The listing builds one solid part. Answer for the finished solid, in the listing's coordinates (mm). Face numbers are marked on the shaded views. A direction names the side the tool comes from. Give positions to 0.01 mm unless a question says otherwise; leave off trailing zeros. Order: outer loops, then holes, each group sorted by start corner. A loop starts at its lowest first (then second) coordinate and runs counter-clockwise, first axis right, second up. Notation, with made-up numbers: (14, 80) -> (46, 80) arc R25 ccw to (46, 110) -> close; hole circle Ø3 at (88.25, 75.5). An arc over 180 degrees is marked (long way). Answer as a JSON object with one key per item and string values. Group by question number.
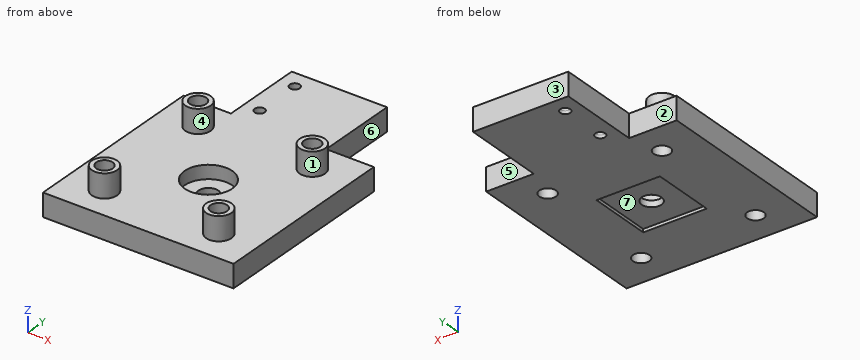
```python
from build123d import *

# Parameters (mm, degrees)
SKETCH1_W           = 38.1
SKETCH1_H           = 76.2
BOSS_EXTRUDE1_DEPTH = 7.9375
SKETCH2_R           = 3.96875
CUT_EXTRUDE1_DEPTH  = 44.330317403
SKETCH4_R           = 9.525
CUT_EXTRUDE2_DEPTH  = 5.3975
SKETCH8_W           = 19.05
SKETCH8_H           = 76.2
BOSS_EXTRUDE5_DEPTH = 7.9375
SKETCH5_R           = 5.08
BOSS_EXTRUDE2_DEPTH = 9.4488
SKETCH6_R           = 3.302
CUT_EXTRUDE3_DEPTH  = 57.617165486
SKETCH7_W           = 38.1
SKETCH7_H           = 33.02
SKETCH7_R           = 2
BOSS_EXTRUDE4_DEPTH = 7.9375
SKETCH9_R           = 3.302
SKETCH9_R_2         = 2
SKETCH9_W           = 25.4
SKETCH9_H           = 25.4
BOSS_EXTRUDE6_DEPTH = 1.27


with BuildPart() as part:
    # Sketch1 → Boss-Extrude1 (new body)
    with BuildSketch(Plane.XY):
        Rectangle(SKETCH1_W, SKETCH1_H)
    extrude(amount=BOSS_EXTRUDE1_DEPTH)

    # Sketch2 → Cut-Extrude1 (cut, through all)
    with BuildSketch(Plane.XY.offset(7.9375)):
        Circle(SKETCH2_R)
    extrude(amount=-CUT_EXTRUDE1_DEPTH, mode=Mode.SUBTRACT)

    # Sketch4 → Cut-Extrude2 (cut)
    with BuildSketch(Plane.XY.offset(7.9375)):
        Circle(SKETCH4_R)
    extrude(amount=-CUT_EXTRUDE2_DEPTH, mode=Mode.SUBTRACT)

    # Sketch8 → Boss-Extrude5 (add)
    with BuildSketch(Plane.XY.offset(7.9375)):
        with Locations((-28.575, 0)):
            Rectangle(SKETCH8_W, SKETCH8_H)
        with Locations((28.575, 0)):
            Rectangle(SKETCH8_W, SKETCH8_H)
    extrude(amount=-BOSS_EXTRUDE5_DEPTH)

    # Sketch5 → Boss-Extrude2 (add)
    with BuildSketch(Plane.XY.offset(7.9375)):
        with Locations(Location((22.86, 25.4, 0), (0, 0, 180))):
            Circle(SKETCH5_R)
        with Locations(Location((-22.86, 25.4, 0), (0, 0, 180))):
            Circle(SKETCH5_R)
    boss_extrude2 = extrude(amount=BOSS_EXTRUDE2_DEPTH)

    # Sketch6 → Cut-Extrude3 (cut, through all)
    with BuildSketch(Plane.XY.offset(17.3863)):
        with Locations((22.86, 25.4)):
            Circle(SKETCH6_R)
        with Locations(Location((-22.86, 25.4, 0), (0, 0, 180))):
            Circle(SKETCH6_R)
    cut_extrude3 = extrude(amount=-CUT_EXTRUDE3_DEPTH, mode=Mode.SUBTRACT)

    # Mirror1: Boss-Extrude2, Cut-Extrude3 across plane
    add(boss_extrude2.mirror(Plane.ZX))
    add(cut_extrude3.mirror(Plane.ZX), mode=Mode.SUBTRACT)

    # Sketch7 → Boss-Extrude4 (add)
    with BuildSketch(Plane.XY.offset(7.9375)):
        with Locations((0, 54.61)):
            Rectangle(SKETCH7_W, SKETCH7_H)
        with Locations((-12.7, 64.135)):
            Circle(SKETCH7_R, mode=Mode.SUBTRACT)
        with Locations(Location((-12.7, 45.085, 0), (0, 0, 180))):
            Circle(SKETCH7_R, mode=Mode.SUBTRACT)
    extrude(amount=-BOSS_EXTRUDE4_DEPTH)

    # Sketch9 → Boss-Extrude6 (add)
    with BuildSketch(Plane(origin=(0, 0, 0), x_dir=(-1, 0, 0), z_dir=(0, 0, -1))):
        Polygon((-19.05, 38.1), (-38.1, 38.1), (-38.1, -38.1), (38.1, -38.1), (38.1, 38.1), (19.05, 38.1), (19.05, 71.12), (-19.05, 71.12), align=None)
        with Locations(Location((-22.86, -25.4, 0), (0, 0, 180))):
            Circle(SKETCH9_R, mode=Mode.SUBTRACT)
        with Locations((22.86, -25.4)):
            Circle(SKETCH9_R, mode=Mode.SUBTRACT)
        with Locations((22.86, 25.4)):
            Circle(SKETCH9_R, mode=Mode.SUBTRACT)
        with Locations(Location((12.7, 64.135, 0), (0, 0, 180))):
            Circle(SKETCH9_R_2, mode=Mode.SUBTRACT)
        with Locations((12.7, 45.085)):
            Circle(SKETCH9_R_2, mode=Mode.SUBTRACT)
        with Locations(Location((-22.86, 25.4, 0), (0, 0, 180))):
            Circle(SKETCH9_R, mode=Mode.SUBTRACT)
        Rectangle(SKETCH9_W, SKETCH9_H, mode=Mode.SUBTRACT)
    extrude(amount=BOSS_EXTRUDE6_DEPTH)


solid = part.part
```
(1) A cutting plane is placed at B-B (x = 0). Determine the outline of the cut face in (y, z) (1 decimal).
(2) A cutting plane is placed at D-D (y = 25.4). Determine the outline of the cut face in (x, z).
(3) For a pull along X with two mould halves and no side action, classify the marked faces 4, 5, 6 and 7 as +X half, -X half, draft (parallel to the pull), parting line (faces both ways), or undercut.
(4) Which of the six approach directions +Z, -Z, +X, -X, +Y, -Y give full straight-line access (tool end or side, diameter ignored) to the marked faces 1, 2 and 3?
(5) A cutting plane is placed at A-A (z = 11.5). Determine the outline of the cut face in (x, y), and give its area (3 significant figures).
(6) A cutting plane is placed at C-C (y = 0). Determine the outline of the cut face in (x, z) (1 decimal).
(7) Find the intervals of material crossed by line 1 along X through (y, z) = (-25, 10.5); line 2 along X through (y, z) = (25.4, 4.5); line 3 along Y through (x, z) = (22.86, 9), in increasing order. Write a range as [from, to].
(8) Flat-ended cylindrical pins translate along their axes: pin 1 Ø21 at (x, y) = (-4, -2) entering from +Z; pin 2 Ø10.5 at (x, y) = (0, 0) entering from +Z; pin 3 Ø4 at (y, z) = (20.5, 15.5) entering from -X. Find the tip coordinate at first contact, or state that the pin passes through.
Check sheet entries:
{
 "1": {"outline": "(-38.1, -1.3) -> (-12.7, -1.3) -> (-12.7, 0) -> (-4, 0) -> (-4, 2.5) -> (-9.5, 2.5) -> (-9.5, 7.9) -> (-38.1, 7.9) -> close; (4, 0) -> (12.7, 0) -> (12.7, -1.3) -> (71.1, -1.3) -> (71.1, 7.9) -> (9.5, 7.9) -> (9.5, 2.5) -> (4, 2.5) -> close"},
 "2": {"outline": "(-38.1, -1.27) -> (-26.16, -1.27) -> (-26.16, 17.39) -> (-27.94, 17.39) -> (-27.94, 7.94) -> (-38.1, 7.94) -> close; (-19.56, -1.27) -> (19.56, -1.27) -> (19.56, 17.39) -> (17.78, 17.39) -> (17.78, 7.94) -> (-17.78, 7.94) -> (-17.78, 17.39) -> (-19.56, 17.39) -> close; (26.16, -1.27) -> (38.1, -1.27) -> (38.1, 7.94) -> (27.94, 7.94) -> (27.94, 17.39) -> (26.16, 17.39) -> close"},
 "3": {"face 4": "undercut", "face 5": "draft", "face 6": "+X half", "face 7": "undercut"},
 "4": {"face 1": "+Z", "face 2": "+Z, -Z, -X, +Y", "face 3": "+Z, -Z, +X, -X, +Y"},
 "5": {"outline": "circle Ø10.16 at (-22.86, -25.4); circle Ø10.16 at (-22.86, 25.4); circle Ø10.16 at (22.86, -25.4); circle Ø10.16 at (22.86, 25.4); hole circle Ø6.6 at (-22.86, -25.4); hole circle Ø6.6 at (-22.86, 25.4); hole circle Ø6.6 at (22.86, -25.4); hole circle Ø6.6 at (22.86, 25.4)", "area": "187 mm2"},
 "6": {"outline": "(-38.1, -1.3) -> (-12.7, -1.3) -> (-12.7, 0) -> (-4, 0) -> (-4, 2.5) -> (-9.5, 2.5) -> (-9.5, 7.9) -> (-38.1, 7.9) -> close; (4, 0) -> (12.7, 0) -> (12.7, -1.3) -> (38.1, -1.3) -> (38.1, 7.9) -> (9.5, 7.9) -> (9.5, 2.5) -> (4, 2.5) -> close"},
 "7": {"line 1": "x = [-27.92, -26.14], [-19.58, -17.8], [17.8, 19.58], [26.14, 27.92]", "line 2": "x = [-38.1, -26.16], [-19.56, 19.56], [26.16, 38.1]", "line 3": "y = [-30.48, -28.7], [-22.1, -20.32], [20.32, 22.1], [28.7, 30.48]"},
 "8": {"pin 1": "stops at z = 7.94", "pin 2": "stops at z = 2.54", "pin 3": "stops at x = -27.03"}
}
